The model under review builds one solid part; all positions refer to its coordinate system, in mm. Coordinates: 2 decimals unless noted, no trailing zeros. Write each loop counter-clockwise with the first axis right and the second up, starting at its lowest first coordinate (ties: lowest second). Pieces come first, ordered by that corner, then holes.
1) Add section D-D, the plane y = 21. State the section outline as (x, z) points.
2) For P1, Ø12, axis at x = -18, y = 21, coming from the +Z side, flat-tipped, find the tip position at first contact; note if it passes through.
3) Add section B-B, the plane z = 319.5. State the section outline as (x, y) points.
4) Add section C-C, the plane y = 79.5. State the section outline as (x, z) points.
5) For line 1 (X direction, y = 35.5, z = -4.5); line 2 (Z direction, x = 235, y = 77.5); line 3 (Z direction, x = -181, y = 98.5), list the stretches that pass through material, from the lowest coordinate up.
6) Add section A-A, the plane x = 198.5. State the section outline as (y, z) points.
Autodesk Inventor part; units mm, degrees
ref_plane "YZ Plane" through (0, 0, 0) normal (1, 0, 0) x (0, 1, 0)
ref_plane "XZ Plane" through (0, 0, 0) normal (0, 1, 0) x (-1, 0, 0)
ref_plane "XY Plane" through (0, 0, 0) normal (0, 0, 1) x (1, 0, 0)
sketch "Sketch1" plane through (0, 0, 0) normal (0, 1, 0) x (-1, 0, 0)
  line L0 (-355.6, 412.75) -> (355.6, 412.75)
  line L1 (355.6, 412.75) -> (355.6, -412.75)
  line L2 (355.6, -412.75) -> (-355.6, -412.75)
  line L3 (-355.6, -412.75) -> (-355.6, 412.75)
  line L4 (-355.6, 412.75) -> (355.6, -412.75) construction
  line L5 (355.6, 412.75) -> (-355.6, -412.75) construction
  line L6 (-426.72, 495.3) -> (426.72, 495.3)
  line L7 (426.72, 495.3) -> (426.72, -495.3)
  line L8 (426.72, -495.3) -> (-426.72, -495.3)
  line L9 (-426.72, -495.3) -> (-426.72, 495.3)
  line L10 (-426.72, 495.3) -> (426.72, -495.3) construction
  line L11 (426.72, 495.3) -> (-426.72, -495.3) construction
  point P0 (0, 0)
  dimension "d0" = 825.5
  dimension "d1" = 711.2
  dimension "d2" = 82.55
extrude "Extrusion1" add sketch "Sketch1" along normal blind 127
fillet "Fillet1" radius 31.75 12 edges at (426.72, 127, 0) (0, 127, 495.3) (-426.72, 127, 0) (0, 127, -495.3) (426.72, 0, 0) (0, 0, 495.3) (0, 0, -495.3) (426.72, 63.5, -495.3) (426.72, 63.5, 495.3) (-426.72, 63.5, -495.3) (-426.72, 0, 0) (-426.72, 63.5, 495.3)
properties part number "bumpers"
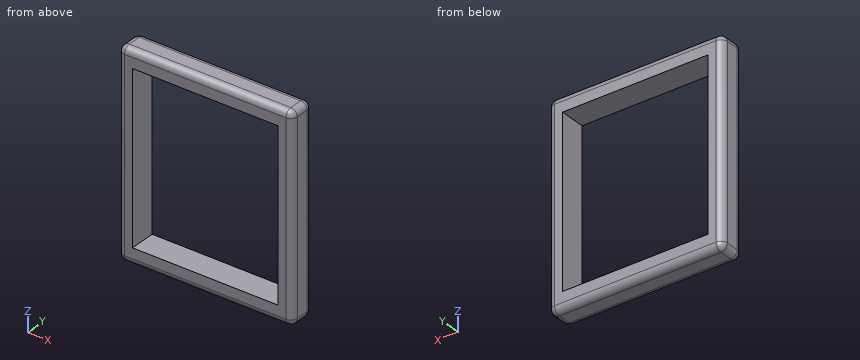
Geometry results:
1. outline: (-424.84, -463.55) arc R29.87 ccw to (-394.97, -493.42) - (394.97, -493.42) arc R29.87 ccw to (424.84, -463.55) - (424.84, 463.55) arc R29.87 ccw to (394.97, 493.42) - (-394.97, 493.42) arc R29.87 ccw to (-424.84, 463.55) - close; hole (-355.6, -412.75) - (355.6, -412.75) - (355.6, 412.75) - (-355.6, 412.75) - close
2. P1: stops at z = 494.94
3. outline: (-426.72, 31.75) arc R31.75 ccw to (-394.97, 0) - (-355.6, 0) - (-355.6, 127) - (-394.97, 127) arc R31.75 ccw to (-426.72, 95.25) - close; (355.6, 0) - (394.97, 0) arc R31.75 ccw to (426.72, 31.75) - (426.72, 95.25) arc R31.75 ccw to (394.97, 127) - (355.6, 127) - close
4. outline: (-426.72, -463.55) arc R31.75 ccw to (-394.97, -495.3) - (394.97, -495.3) arc R31.75 ccw to (426.72, -463.55) - (426.72, 463.55) arc R31.75 ccw to (394.97, 495.3) - (-394.97, 495.3) arc R31.75 ccw to (-426.72, 463.55) - close; hole (-355.6, -412.75) - (355.6, -412.75) - (355.6, 412.75) - (-355.6, 412.75) - close
5. line 1: x = -426.72 to -355.6, 355.6 to 426.72
5. line 2: z = -495.3 to -412.75, 412.75 to 495.3
5. line 3: z = -495.13 to -412.75, 412.75 to 495.13
6. outline: (0, -463.55) arc R31.75 ccw to (31.75, -495.3) - (95.25, -495.3) arc R31.75 ccw to (127, -463.55) - (127, -412.75) - (0, -412.75) - close; (0, 412.75) - (127, 412.75) - (127, 463.55) arc R31.75 ccw to (95.25, 495.3) - (31.75, 495.3) arc R31.75 ccw to (0, 463.55) - close
